```python
from build123d import *

# Parameters (mm, degrees)
F0_W     = 5
F0_H     = 5
F1_DEPTH = 2
F0_R     = 1.25
F2_DEPTH = 8
F3_DEPTH = 6
F5_R     = 3
F6_DEPTH = 50
F7_R     = 1.99999


# Not quite as in the source:
# - a fillet or chamfer is up to 0.001 mm smaller than in the source, because OpenCascade refuses the exact size


with BuildPart() as f1:
    # F0 (on Top) → F1 (new body)
    with BuildSketch(Plane.XY):
        with Locations((-33.5, 13)):
            Rectangle(F0_W, F0_H)
        with BuildLine():
            Line((-31, -15.5), (28, -15.5))
            ThreePointArc((28, -15.5), (30.1213203436, -14.6213203436), (31, -12.5))
            Line((31, -12.5), (31, -5))
            Line((31, -5), (31, 5))
            Line((31, 5), (31, 12.5))
            ThreePointArc((31, 12.5), (30.1213203436, 14.6213203436), (28, 15.5))
            Line((28, 15.5), (-31, 15.5))
            Line((-31, 15.5), (-31, 10.5))
            Line((-31, 10.5), (-31, -10.5))
            Line((-31, -10.5), (-31, -15.5))
        make_face()
        with Locations((-33.5, -13)):
            Rectangle(F0_W, F0_H)
    extrude(amount=F1_DEPTH)

    # F0 (on Top) → F2 (join)
    with BuildSketch(Plane.XY):
        with BuildLine():
            Line((31, 5), (31, -5))
            Line((31, -5), (36, -5))
            ThreePointArc((36, -5), (39.5355339059, -3.5355339059), (41, 0))
            ThreePointArc((41, 0), (39.5355339059, 3.5355339059), (36, 5))
            Line((36, 5), (31, 5))
        make_face()
        with Locations((36, 0)):
            Circle(F0_R, mode=Mode.SUBTRACT)
        with BuildLine():
            Line((-31, -15.5), (28, -15.5))
            ThreePointArc((28, -15.5), (30.1213203436, -14.6213203436), (31, -12.5))
            Line((31, -12.5), (31, -5))
            Line((31, -5), (31, 5))
            Line((31, 5), (31, 12.5))
            ThreePointArc((31, 12.5), (30.1213203436, 14.6213203436), (28, 15.5))
            Line((28, 15.5), (-31, 15.5))
            Line((-31, 15.5), (-31, 10.5))
            Line((-31, 10.5), (-31, -10.5))
            Line((-31, -10.5), (-31, -15.5))
        make_face()
    extrude(amount=F2_DEPTH)

    # F0 (on Top) → F3 (cut)
    with BuildSketch(Plane.XY):
        with BuildLine():
            Line((31, 5), (31, -5))
            Line((31, -5), (36, -5))
            ThreePointArc((36, -5), (39.5355339059, -3.5355339059), (41, 0))
            ThreePointArc((41, 0), (39.5355339059, 3.5355339059), (36, 5))
            Line((36, 5), (31, 5))
        make_face()
        with Locations((36, 0)):
            Circle(F0_R, mode=Mode.SUBTRACT)
    extrude(amount=F3_DEPTH, mode=Mode.SUBTRACT)

    # F5
    f5_edges = [f1.edges().sort_by_distance(p)[0] for p in [
        (-31, 15.5, 5),
        (-31, -15.5, 5),
    ]]
    fillet(f5_edges, radius=F5_R)

    # F4 (on face) → F6 (cut)
    with BuildSketch(Plane.XZ.offset(15.5)):
        with BuildLine():
            Line((8, 8), (-21.3, 8))
            add(Edge.make_bspline(
                [(-21.3, 8), (-18.6027030945, 5.1925020669), (-11.9176320955, 0.5356481102), (0.5768376855, 4.4751283983), (8, 8)],
                knots=[0, 0, 0, 0, 0.4179419715, 1, 1, 1, 1], degree=3))
        make_face()
    extrude(amount=-F6_DEPTH, mode=Mode.SUBTRACT)

    # F7 (radius 2 in the source; OpenCascade refuses exactly that, so slightly less here)
    f7_edges = [f1.edges().sort_by_distance(p)[0] for p in [
        (33.5, -5, 8),
        (30.12132, -14.62132, 8),
        (-7.010651, -15.5, 2.945097),
        (8, 0, 8),
        (-7.010651, 15.5, 2.945097),
        (-21.3, 0, 8),
        (33.5, 5, 8),
        (31, 8.75, 8),
        (30.12132, 14.62132, 8),
        (-24.65, -15.5, 8),
        (-30.12132, -14.62132, 8),
        (-31, 0, 8),
        (-30.12132, 14.62132, 8),
        (-24.65, 15.5, 8),
        (18, -15.5, 8),
        (31, -8.75, 8),
        (41, 0, 8),
        (18, 15.5, 8),
    ]]
    fillet(f7_edges, radius=F7_R)


solid = f1.part
```
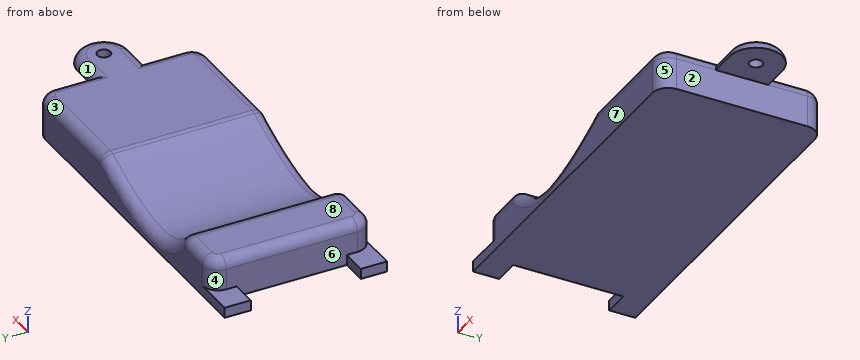
Part model, mm, in its own coordinate system. Face numbers are marked on the shaded views. A direction names the side the tool comes from. Round coordinates to 2 decimals unless told otherwise and drop trailing zeros. Use CSV: the item, a comma, the result in double quotes. Start each with the question number.
1) Wall check: L1, parallel to X at y = -0.5, z = 7.5; L2, parallel to X at y = 1, z = 6.25; L3, parallel to Y at x = 36, z = 6.55. Give the ranges that are in metal, low to high. Write a range as [from, to].
2) Pull direction Y, two halves, no side cores. Call the marked faces 6, 7 and 8: +Y half, -Y half, draft (parallel to the pull), parting line (faces both ways), or undercut.
3) Drop flat-ended pins along their axis: P1, Ø5.5, axis at x = -32, y = -13.5, coming from the +Z side; P2, Ø1.5, axis at x = -32.5, y = 13, coming from the +Z side; P3, Ø3, axis at y = 1, z = 2.5, coming from the -X side. Give the stop position or say it passes through.
4) Which spindle directions (+Z, -Z, +X, -X, +Y, -Y) get a long thin tool onto all of the face, cutting with end or side? Do the marked faces 1, 2, 3, 4 and 5. Say none if no direction does.
Determined:
1,L1,"x = [-30.32, -20.81], [6.93, 34.85], [37.15, 40.29]"
1,L2,"x = [-30.98, -19.46], [4.07, 35.25], [36.75, 40.88]"
1,L3,"y = [-4.92, -1.25], [1.25, 4.92]"
2,face 6,"undercut"
2,face 7,"-Y half"
2,face 8,"draft"
3,P1,"stops at z = 7.96"
3,P2,"stops at z = 2"
3,P3,"stops at x = -31"
4,face 1,"+Z, +X, +Y"
4,face 2,"-Z, +X, +Y, -Y"
4,face 3,"+Z, +X, -X, +Y"
4,face 4,"+Z, -X, +Y"
4,face 5,"+Z, -Z, +X, -Y"
